Geometry: see drawing. Coordinates: mm, zero at the bounding-box minimum. A direction names the side the tool comes from. Coordinates: 2 decimals unless noted, no trailing zeros. Loops run counter-clockwise (first coordinate to the right, second up) from the corner with the lowest first, then second, coordinate; pieces in that order, holes last. Notation, with made-up numbers: (70.25, 72.5) - (85.25, 72.5) arc R14 cw to (85.25, 83.5) - close; hole circle Ø7 at (84, 34). An arc over 180 degrees is marked (long way). Answer in a Markdown table with one row per item.
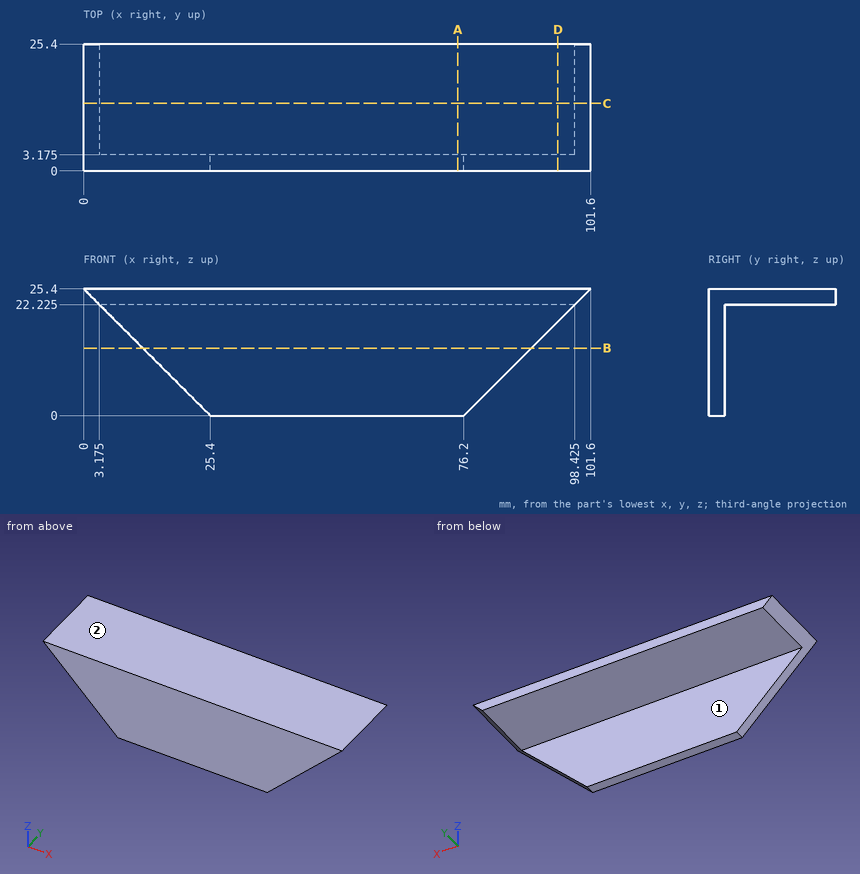
(1) Access query for the marked faces 1 and 2. Directions: +Z, -Z, +X, -X, +Y, -Y. A direction counts if a zero-diameter tool reaches every point of the face in a straight line with its end or side. Return the directions, or none.
Verdict:
| item | result |
|---|---|
| face 1 | -Z, +X, -X, +Y |
| face 2 | +Z, +X, -X, +Y, -Y |
(2) Cut plane A-A on x = 75. Output: boundary loops of the cut face in (y, z) (3 decimals).
Verdict:
| item | result |
|---|---|
| outline | (0, 0) - (3.175, 0) - (3.175, 22.225) - (25.4, 22.225) - (25.4, 25.4) - (0, 25.4) - close |
(3) Ray query, probe 1 along Z at (x, y) = (21, 17.5) (3 decimals); probe 2 along Y at (x, z) = (42.5, 19) (3 decimals); probe 3 along X at (y, z) = (7, 24.25). Return the intervals inside material, ascending.
Verdict:
| item | result |
|---|---|
| probe 1 | z = 22.225 to 25.4 |
| probe 2 | y = 0 to 3.175 |
| probe 3 | x = 1.15 to 100.45 |
(4) Cut plane D-D on x = 95. Output: boundary loops of the cut face in (y, z) (3 decimals).
Verdict:
| item | result |
|---|---|
| outline | (0, 18.8) - (3.175, 18.8) - (3.175, 22.225) - (25.4, 22.225) - (25.4, 25.4) - (0, 25.4) - close |
(5) Cut plane C-C on y = 13.5. Output: boundary loops of the cut face in (x, z) (3 decimals), then the cut area to 4 significant figures.
Verdict:
| item | result |
|---|---|
| outline | (0, 25.4) - (3.175, 22.225) - (98.425, 22.225) - (101.6, 25.4) - close |
| area | 312.5 mm² |
(6) Cut plane B-B on z = 13.5. Output: boundary loops of the cut face in (x, y) (3 decimals), then the cut area to 3 significant figures.
Verdict:
| item | result |
|---|---|
| outline | (11.9, 0) - (89.7, 0) - (89.7, 3.175) - (11.9, 3.175) - close |
| area | 247 mm² |
(7) First-contact query: pin 1 Ø5 at (x, z) = (50, 16) entering from +Y (3 decimals); pin 2 Ø1.5 at (y, z) = (22.5, 22) entering from -X; pin 3 Ø6.5 at (x, y) = (73, 10) entering from -Z (3 decimals). Flat tips, straight axial feed; report the tip coordinate or a pass-through.
Verdict:
| item | result |
|---|---|
| pin 1 | stops at y = 3.175 |
| pin 2 | stops at x = 2.65 |
| pin 3 | stops at z = 22.225 |
